```python
from build123d import *

# Parameters (mm, degrees)
F1_DEPTH       = 25
F3_D           = 3.2639
F3_CSINK_D     = 6.477
F3_CSINK_ANGLE = 82


with BuildPart() as f1:
    # F0 (on Top) → F1 (new body)
    with BuildSketch(Plane.XY):
        Polygon((-29.003669071, 6), (-29.003669071, -21.425), (-23.003669071, -21.425), (-23.003669071, 0), (-5.5934852733, 0), (-5.5934852733, 6), align=None)
    extrude(amount=F1_DEPTH)

    # F3 (through all)
    with Locations(Plane(origin=(-29.003669071, 0, 0), x_dir=(0, -1, 0), z_dir=(-1, 0, 0))):
        with Locations((16.4713294148, 12.5)):
            CounterSinkHole(F3_D / 2, F3_CSINK_D / 2, counter_sink_angle=F3_CSINK_ANGLE)


solid = f1.part
```
Here's how the part is built. I have some questions about the finished solid (model axes, mm). A direction names the side the tool comes from. Coordinates: 2 decimals unless noted, no trailing zeros. Order: outer loops, then holes, each group sorted by start corner. A loop starts at its lowest first (then second) coordinate and runs counter-clockwise, first axis right, second up. Notation, with made-up numbers: (-26.5, -35.5) -> (1.5, -35.5) arc R13 ccw to (1.5, -23.5) -> close; hole circle Ø5 at (73.5, 49). An arc over 180 degrees is marked (long way). Return JSON: item names as keys, results as strings.
1) If we section it at C-C on x = -11.5: List the corners of the cut face in (y, z) for me, plus the area to 3 significant figures.
Conclusion:
{"outline": "(0, 0) -> (6, 0) -> (6, 25) -> (0, 25) -> close", "area": "150 mm²"}
2) I'm going to push flat-ended pins straight in: P1, Ø4, axis at y = -16.47, z = 12.5, coming from the -X side; P2, Ø6.5, axis at y = -11, z = 15, coming from the +X side. Where does each tip first touch, or does it pass through?
Conclusion:
{"P1": "stops at x = -27.58", "P2": "stops at x = -23"}
3) If we section it at D-D on y = -2: List the corners of the cut face in (x, z) for me.
Conclusion:
{"outline": "(-29, 0) -> (-23, 0) -> (-23, 25) -> (-29, 25) -> close"}
4) Thinking about a two-plate mould opening in Z: for faces 1 (the cylindrical face through (-25.051, -14.915, 12.99)), 2 (the flat face through (-25, -1, 0)), 3 (the flat face through (-29.004, -8, 12)), which applies, +Z half, -Z half, draft (parallel to the pull), parting line (faces both ways), or undercut?
Conclusion:
{"face 1": "undercut", "face 2": "-Z half", "face 3": "draft"}
5) On a 3-axis mill with a long thin cutter (end or side, diameter ignored), from which of +Z, -Z, +X, -X, +Y, -Y can I reach the whole of each face in a straight line? I mean faces 4 (the flat face through (-26, -21.425, 12)), 5 (the flat face through (-14, 0, 12)). Say none if no direction works.
Conclusion:
{"face 4": "+Z, -Z, +X, -X, -Y", "face 5": "+Z, -Z, +X, -Y"}
6) If we section it at B-B on z = 6.5: List the corners of the cut face in (x, y) for me (3 decimals), plus the area to 3 significant figures.
Conclusion:
{"outline": "(-29.004, -21.425) -> (-23.004, -21.425) -> (-23.004, 0) -> (-5.593, 0) -> (-5.593, 6) -> (-29.004, 6) -> close", "area": "269 mm²"}
7) If I drill on probe 1 along Y at (x, z) = (-24.6, 12.5) (3 decimals); probe 2 along X at (y, z) = (-15.75, 6.25); probe 3 along Y at (x, z) = (-10, 23.5), over which ranges is the centre line in solid material (lowest first)?
Conclusion:
{"probe 1": "y = -21.425 to -18.103, -14.839 to 6", "probe 2": "x = -29 to -23", "probe 3": "y = 0 to 6"}
8) If we section it at A-A on z = 12.5: List the corners of the cut face in (x, y) for me (3 decimals), plus the area to 3 significant figures.
Conclusion:
{"outline": "(-29.004, -21.425) -> (-23.004, -21.425) -> (-23.004, -18.103) -> (-27.156, -18.103) -> (-29.004, -19.71) -> close; (-29.004, -13.233) -> (-27.156, -14.839) -> (-23.004, -14.839) -> (-23.004, 0) -> (-5.593, 0) -> (-5.593, 6) -> (-29.004, 6) -> close", "area": "246 mm²"}
